from build123d import *

# Parameters (mm, degrees)
SKETCH1_W                         = 44.45
SKETCH1_H                         = 44.45
BOSS_EXTRUDE1_DEPTH               = 19.05
F_12_28_TAPPED_HOLE1_D            = 4.6228
F_12_28_TAPPED_HOLE1_DEPTH        = 11.43
F_12_28_TAPPED_HOLE1_CSINK_D      = 6.7564
F_12_28_TAPPED_HOLE1_CSINK_ANGLE  = 100
F_12_28_TAPPED_HOLE1_TIP          = 1.388829235
PIPE_TAP_DRILL_FOR_1_8_TAP1_D     = 8.4328
PIPE_TAP_DRILL_FOR_1_8_TAP1_DEPTH = 35.052
PIPE_TAP_DRILL_FOR_1_8_TAP1_TIP   = 2.533468714
F_10_32_TAPPED_HOLE1_D            = 4.0386
F_3_8_24_TAPPED_HOLE1_D           = 8.4328
F_3_8_24_TAPPED_HOLE1_DEPTH       = 9.652
F_3_8_24_TAPPED_HOLE1_TIP         = 2.533468714


with BuildPart() as part:
    # Sketch1 → Boss-Extrude1 (new body)
    with BuildSketch(Plane.XY):
        Rectangle(SKETCH1_W, SKETCH1_H)
    extrude(amount=BOSS_EXTRUDE1_DEPTH)

    # #12-28 Tapped Hole1
    with Locations(Plane.XY.offset(19.05)):
        with Locations((-9.525, 0)):
            CounterSinkHole(F_12_28_TAPPED_HOLE1_D / 2, F_12_28_TAPPED_HOLE1_CSINK_D / 2, depth=F_12_28_TAPPED_HOLE1_DEPTH, counter_sink_angle=F_12_28_TAPPED_HOLE1_CSINK_ANGLE)
            with Locations((0, 0, -(F_12_28_TAPPED_HOLE1_DEPTH + F_12_28_TAPPED_HOLE1_TIP / 2))):  # 118° drill point
                Cone(0, F_12_28_TAPPED_HOLE1_D / 2, F_12_28_TAPPED_HOLE1_TIP, mode=Mode.SUBTRACT)

    # Pipe Tap Drill for 1/8 Tap1
    with Locations(Plane(origin=(22.225, 0, 0), x_dir=(0, 0, -1), z_dir=(1, 0, 0))):
        with Locations((-7.9375, 7.9375), (-7.9375, -7.9375)):
            Hole(PIPE_TAP_DRILL_FOR_1_8_TAP1_D / 2, depth=PIPE_TAP_DRILL_FOR_1_8_TAP1_DEPTH)
            with Locations((0, 0, -(PIPE_TAP_DRILL_FOR_1_8_TAP1_DEPTH + PIPE_TAP_DRILL_FOR_1_8_TAP1_TIP / 2))):  # 118° drill point
                Cone(0, PIPE_TAP_DRILL_FOR_1_8_TAP1_D / 2, PIPE_TAP_DRILL_FOR_1_8_TAP1_TIP, mode=Mode.SUBTRACT)

    # #10-32 Tapped Hole1 (through all)
    with Locations(Plane.XY.offset(19.05)):
        with Locations((9.525, 15.875), (9.525, -15.875)):
            Hole(F_10_32_TAPPED_HOLE1_D / 2)

    # 3/8-24 Tapped Hole1
    with Locations(Plane(origin=(0, 0, 0), x_dir=(-1, 0, 0), z_dir=(0, 0, -1))):
        with Locations((9.525, 0)):
            Hole(F_3_8_24_TAPPED_HOLE1_D / 2, depth=F_3_8_24_TAPPED_HOLE1_DEPTH)
            with Locations((0, 0, -(F_3_8_24_TAPPED_HOLE1_DEPTH + F_3_8_24_TAPPED_HOLE1_TIP / 2))):  # 118° drill point
                Cone(0, F_3_8_24_TAPPED_HOLE1_D / 2, F_3_8_24_TAPPED_HOLE1_TIP, mode=Mode.SUBTRACT)


solid = part.part
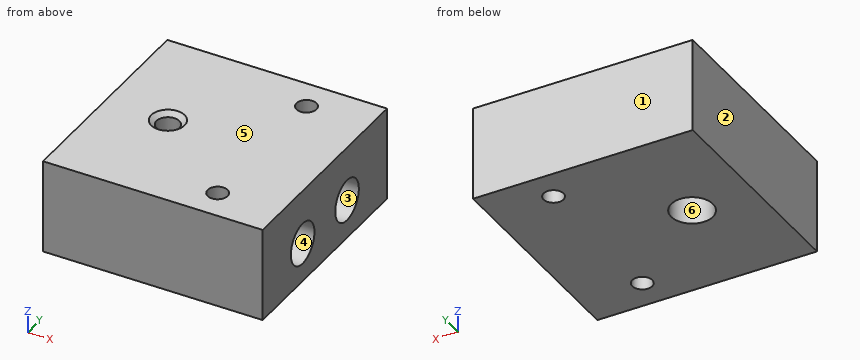
Could you check a few things on this model? Use its own coordinates, in mm. Face numbers are marked on the shaded views. A direction names the side the tool comes from. Give positions to 0.01 mm unless a question says otherwise; leave off trailing zeros. Order: outer loops, then holes, each group sorted by start corner. A loop starts at its lowest first (then second) coordinate and runs counter-clockwise, first axis right, second up. Notation, with made-up numbers: (88.5, 26) - (146.5, 26) arc R20 cw to (146.5, 48) - close; hole circle Ø11 at (89.25, 26.25). An arc over 180 degrees is marked (long way). Return JSON: item names as keys, results as strings. Group by question number.
Q1. Which directions (+Z, -Z, +X, -X, +Y, -Y) give clear straight access to the entire face, cutting with the end or side of a thin tool? Please do the marked faces 4, 5 and 6.
Q2. Suppose I cut it at C-C, the plane x = 2. State how many separate pieces and enclosed holes the cut face has, and give its area (3 significant figures).
Q3. Please list where these lines run through material, in increasing order: line 1 along X through (y, z) = (0, 7.75) (3 decimals); line 2 along Y through (x, z) = (19, 6.5) (3 decimals); line 3 along Y through (x, z) = (19, 11.75) (3 decimals). Write a range as [from, to].
Q4. Suppose I cut it at A-A, the plane y = 0. Please give me the cut outline in (x, z) (3 decimals), and give its area (3 significant figures).
Q5. Thinking about a two-plate mould opening in Y: for the marked faces 1, 2 and 3, which applies, pulls with the +Y half, pulls with the -Y half, needs draft (parallel to the pull), parting line crosses it, or undercut?
Q6. Suppose I cut it at B-B, the plane z = 1. Please give me the cut outline in (x, y) (3 decimals).
Q7. Will these pins go through, and if not, where does the flat tip stop? pin 1 Ø6.5 at (x, y) = (9.525, 15.875) entering from +Z; pin 2 Ø6.5 at (y, z) = (7.94, 7.94) entering from +X.
Resolved:
{
 "1": {"face 4": "+X", "face 5": "+Z, +X, -X, +Y, -Y", "face 6": "-Z"},
 "2": {"separate pieces": "1", "enclosed holes": "2", "area": "735 mm2"},
 "3": {"line 1": "x = [-22.225, -13.741], [-5.309, 22.225]", "line 2": "y = [-22.225, -11.901], [-3.974, 3.974], [11.901, 22.225]", "line 3": "y = [-22.225, -9.738], [-6.137, 6.137], [9.738, 22.225]"},
 "4": {"outline": "(-22.225, 0) - (-13.741, 0) - (-13.741, 9.652) - (-11.836, 10.797) - (-11.836, 18.155) - (-12.903, 19.05) - (-22.225, 19.05) - close; (-7.214, 10.797) - (-5.309, 9.652) - (-5.309, 0) - (22.225, 0) - (22.225, 19.05) - (-6.147, 19.05) - (-7.214, 18.155) - close", "area": "719 mm2"},
 "5": {"face 1": "pulls with the +Y half", "face 2": "needs draft", "face 3": "undercut"},
 "6": {"outline": "(-22.225, -22.225) - (22.225, -22.225) - (22.225, 22.225) - (-22.225, 22.225) - close; hole circle Ø8.433 at (-9.525, 0); hole circle Ø4.039 at (9.525, -15.875); hole circle Ø4.039 at (9.525, 15.875)"},
 "7": {"pin 1": "stops at z = 19.05", "pin 2": "stops at x = -13.41"}
}
